Geometry check sheet. Reference: drawing and pictorial views, mm from the part's lowest x, y, z. A direction names the side the tool comes from. Give positions to 0.01 mm unless a question says otherwise; leave off trailing zeros. Loops run counter-clockwise (first coordinate to the right, second up) from the corner with the lowest first, then second, coordinate; pieces in that order, holes last. Notation, with made-up numbers: (-31.5, 50) - (-15.5, 50) arc R14 cw to (-15.5, 73) - close; hole circle Ø6 at (-26.75, 79.25). An arc over 180 degrees is marked (long way). Answer in a Markdown table with one row per item. Add a question column.
(1) Thickness scan on L1, parallel to Y at x = 2.5, z = 0.85; L2, parallel to Z at x = 4, y = 12; L3, parallel to X at y = 14.75, z = 5.25. Record the ranges inside material, lowest first.
(2) Sectioned sample at D-D on y = 2. Enter the section's corners in (x, z).
(3) Draft check along Z on the marked faces 1, 2 and 3. Enter one of: released by +Z, released by -Z, zero draft, split by the parting line, or undercut.
(4) Go/stop test with flat-tipped pins: P1, Ø4, axis at x = 15, y = 8, coming from the -Z side; P2, Ø1.5, axis at x = 21.22, y = 8, coming from the -Z side. Record where each tip stops, or that it passes through.
(5) Sectioned sample at A-A on x = 15. Enter the section's corners in (y, z), then the cut area to 3 significant figures.
(6) Set-up check for the marked faces 4 and 5: record each of +Z, -Z, +X, -X, +Y, -Y from which the full face is reachable in a straight line by a thin tool's end or side.
(7) Sectioned sample at B-B on z = 0.75. Enter the section's corners in (x, y), then the cut area to 3 significant figures.
(8) Sectioned sample at C-C on x = 2.5. Enter the section's corners in (y, z), then the cut area to 3 significant figures.
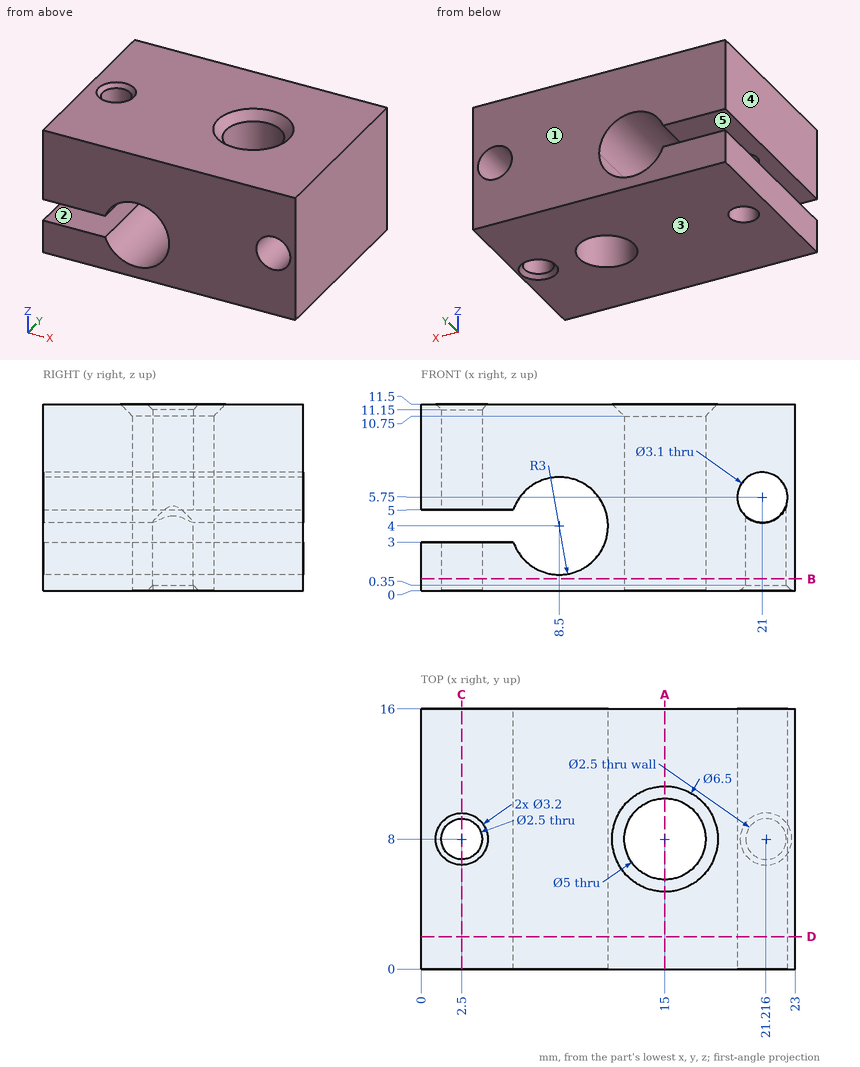
Reply:
| question | item | result |
|---|---|---|
| 1 | L1 | 0 to 6.75, 9.25 to 16 |
| 1 | L2 | 0 to 3, 5 to 11.5 |
| 1 | L3 | 0 to 5.77, 11.23 to 19.53, 22.47 to 23 |
| 2 | outline | (0, 0) - (23, 0) - (23, 11.5) - (0, 11.5) - (0, 5) - (5.67, 5) arc R3 cw (long way) to (5.67, 3) - (0, 3) - close; hole circle Ø3.1 at (21, 5.75) |
| 3 | face 1 | zero draft |
| 3 | face 2 | undercut |
| 3 | face 3 | released by -Z |
| 4 | P1 | through |
| 4 | P2 | z = 6.96 |
| 5 | outline | (0, 0) - (5.5, 0) - (5.5, 10.75) - (4.75, 11.5) - (0, 11.5) - close; (10.5, 0) - (16, 0) - (16, 11.5) - (11.25, 11.5) - (10.5, 10.75) - close |
| 5 | area | 126 mm^2 |
| 6 | face 4 | +Z, -Z, -X, +Y, -Y |
| 6 | face 5 | -X, +Y, -Y |
| 7 | outline | (0, 0) - (23, 0) - (23, 16) - (0, 16) - close; hole circle Ø2.5 at (2.5, 8); hole circle Ø5 at (15, 8); hole circle Ø2.5 at (21.22, 8) |
| 7 | area | 339 mm^2 |
| 8 | outline | (0, 0) - (6.75, 0) - (6.75, 3) - (0, 3) - close; (0, 5) - (6.75, 5) - (6.75, 11.15) - (6.4, 11.5) - (0, 11.5) - close; (9.25, 0) - (16, 0) - (16, 3) - (9.25, 3) - close; (9.25, 5) - (16, 5) - (16, 11.5) - (9.6, 11.5) - (9.25, 11.15) - close |
| 8 | area | 128 mm^2 |
